```python
from build123d import *

# Parameters (mm, degrees)
SKETCH1_R           = 40
BOSS_EXTRUDE1_DEPTH = 5
SKETCH2_R           = 11
BOSS_EXTRUDE2_DEPTH = 5
SKETCH3_R           = 5
CUT_EXTRUDE1_DEPTH  = 58.445626465
SKETCH4_R           = 4
CUT_EXTRUDE2_DEPTH  = 57.789083458


with BuildPart() as part:
    # Sketch1 → Boss-Extrude1 (new body)
    with BuildSketch(Plane(origin=(0, 0, 0), x_dir=(1, 0, 0), z_dir=(0, 1, 0))):
        with Locations(Location((0, 0, 0), (0, 0, 270))):
            Circle(SKETCH1_R)
    extrude(amount=BOSS_EXTRUDE1_DEPTH)

    # Sketch2 → Boss-Extrude2 (add)
    with BuildSketch(Plane.XZ):
        with Locations(Location((0, 0, 0), (0, 0, 270))):
            Circle(SKETCH2_R)
    extrude(amount=BOSS_EXTRUDE2_DEPTH)

    # Sketch3 → Cut-Extrude1 (cut, through all)
    with BuildSketch(Plane.XZ.offset(5)):
        with Locations(Location((0, 0, 0), (0, 0, 270))):
            Circle(SKETCH3_R)
    extrude(amount=-CUT_EXTRUDE1_DEPTH, mode=Mode.SUBTRACT)

    # Sketch4 → Cut-Extrude2 (cut, through all)
    with BuildSketch(Plane.XZ):
        with Locations(Location((32, 0, 0), (0, 0, 270))):
            Circle(SKETCH4_R)
    extrude(amount=-CUT_EXTRUDE2_DEPTH, mode=Mode.SUBTRACT)


solid = part.part
```
Build history of the part. All positions in model axes, mm. A direction names the side the tool comes from. Give positions to 0.01 mm unless a question says otherwise; leave off trailing zeros. Loops run counter-clockwise (first coordinate to the right, second up) from the corner with the lowest first, then second, coordinate; pieces in that order, holes last. Notation, with made-up numbers: (66.5, -34.75) -> (75.5, -34.75) arc R19 cw to (75.5, -6.75) -> close; hole circle Ø1 at (2, -28.5). An arc over 180 degrees is marked (long way). One line per question, with ' | ' between items. Start each with the question number.
1) 3-axis set-ups, long thin cutter, end or side, ignore diameter. For faces 1 (the flat face through (-5, -5, -2)), 2 (the flat face through (-8, 0, 8)): which of +Z, -Z, +X, -X, +Y, -Y reach the whole face in a straight line?
2) Probe L1, parallel to Y at x = -17, z = -24.5; L2, parallel to X at y = -2.25, z = 0; L3, parallel to Z at x = 3, y = 1. List the from-to ranges inside material, lowest first.
3) Cut at D-D (y = -4). Give the cut face in (x, z).
4) Cut at B-B (x = 32). Give the cut face in (y, z), plus the area to 3 significant figures.
5) Cut at A-A (z = 0). Give the cut face in (x, y).
6) Cut at C-C (x = 0). Give the cut face in (y, z), plus the area to 3 significant figures.
7) Pin check, flat tips, straight feed: pin 1 (8 mm diameter, centred on x = 0, z = 0, fed in from -Y); pin 2 (24 mm diameter, centred on x = 9, z = 10, fed in from -Y); pin 3 (3 mm diameter, centred on y = 0, z = -11.5, fed in from -X); pin 4 (6 mm diameter, centred on x = 9, y = -2, fed in from +Z). Stop position of each tip, or through.
Return value:
1) face 1: +Z, -Z, +X, -X, -Y | face 2: -Y
2) L1: 0 to 5 | L2: -11 to -5, 5 to 11 | L3: -39.89 to -4, 4 to 39.89
3) outline: circle Ø22 at (0, 0); hole circle Ø10 at (0, 0)
4) outline: (0, -24) -> (5, -24) -> (5, -4) -> (0, -4) -> close; (0, 4) -> (5, 4) -> (5, 24) -> (0, 24) -> close | area: 200 mm^2
5) outline: (-40, 0) -> (-11, 0) -> (-11, -5) -> (-5, -5) -> (-5, 5) -> (-40, 5) -> close; (5, -5) -> (11, -5) -> (11, 0) -> (28, 0) -> (28, 5) -> (5, 5) -> close; (36, 0) -> (40, 0) -> (40, 5) -> (36, 5) -> close
6) outline: (-5, -11) -> (0, -11) -> (0, -40) -> (5, -40) -> (5, -5) -> (-5, -5) -> close; (-5, 5) -> (5, 5) -> (5, 40) -> (0, 40) -> (0, 11) -> (-5, 11) -> close | area: 410 mm^2
7) pin 1: through | pin 2: y = -5 | pin 3: x = -38.73 | pin 4: z = 39.42
